Autodesk Inventor part; units mm, degrees
ref_plane "YZ Plane" through (0, 0, 0) normal (1, 0, 0) x (0, 1, 0)
ref_plane "XZ Plane" through (0, 0, 0) normal (0, 1, 0) x (-1, 0, 0)
ref_plane "XY Plane" through (0, 0, 0) normal (0, 0, 1) x (1, 0, 0)
sketch "Sketch1" plane through (0, 0, 0) normal (0, 0, 1) x (1, 0, 0)
  line L0 (0, 10.2918) -> (25, 10.2918)
  line L1 (25, 10.2918) -> (25, 0.2918)
  line L2 (25, 0.2918) -> (0, 0.2918)
  line L3 (0, 0.2918) -> (0, 10.2918)
  line L4 (2, 0.2918) -> (10, 0.2918)
  line L5 (10, 0.2918) -> (10, 3.2918)
  line L6 (10, 3.2918) -> (2, 3.2918)
  line L7 (2, 3.2918) -> (2, 0.2918)
  line L8 (0, 5.2918) -> (25, 5.2918) construction
  line L9 (12.5, 10.2918) -> (12.5, 0.2918) construction
  line L10 (23, 0.2918) -> (15, 0.2918)
  line L11 (15, 0.2918) -> (15, 3.2918)
  line L12 (15, 3.2918) -> (23, 3.2918)
  line L13 (23, 3.2918) -> (23, 0.2918)
  line L14 (2, 10.2918) -> (10, 10.2918)
  line L15 (10, 10.2918) -> (10, 7.2918)
  line L16 (10, 7.2918) -> (2, 7.2918)
  line L17 (2, 7.2918) -> (2, 10.2918)
  line L18 (23, 10.2918) -> (15, 10.2918)
  line L19 (15, 10.2918) -> (15, 7.2918)
  line L20 (15, 7.2918) -> (23, 7.2918)
  line L21 (23, 7.2918) -> (23, 10.2918)
  point P0 (0, 0)
  dimension "d0" = 25
  dimension "d1" = 10
  dimension "d2" = 3
  dimension "d3" = 2
  dimension "d4" = 8
extrude "Extrusion1" add sketch "Sketch1" along normal blind 3 contours L0 L17 L16 L15 L19 L20 L21 L1 L2 L13 L12 L11 L5 L6 L7 L3
properties part number "techoProctetorSensorHal"
Geometry check sheet. Reference: the model listing, model coordinates, mm. A direction names the side the tool comes from. Give positions to 0.01 mm unless a question says otherwise; leave off trailing zeros. Loops run counter-clockwise (first coordinate to the right, second up) from the corner with the lowest first, then second, coordinate; pieces in that order, holes last. Notation, with made-up numbers: M 22.5,11.25 L 37.5,11.25 A28 ccw 37.5,39.25 Z; hole C 11,78 d7. An arc over 180 degrees is marked long. Write each question's results on one line, items separated by ' | '.
1) Thickness scan on line 1 (X direction, y = 7.5, z = 2.7); line 2 (Y direction, x = 18, z = 2.05). Record the ranges inside material, lowest first.
Answers follow:
line 1: 0 to 2, 10 to 15, 23 to 25 | line 2: 3.29 to 7.29
2) Section check C-C, the plane x = 16. Record the boundary of the cut face in (y, z), plus the area to 3 significant figures.
Answers follow:
outline: M 3.29,0 L 7.29,0 L 7.29,3 L 3.29,3 Z | area: 12.0 mm2
3) Section check B-B, the plane z = 1.5. Record the boundary of the cut face in (x, y), plus the area to 3 significant figures.
Answers follow:
outline: M 0,0.29 L 2,0.29 L 2,3.29 L 10,3.29 L 10,0.29 L 15,0.29 L 15,3.29 L 23,3.29 L 23,0.29 L 25,0.29 L 25,10.29 L 23,10.29 L 23,7.29 L 15,7.29 L 15,10.29 L 10,10.29 L 10,7.29 L 2,7.29 L 2,10.29 L 0,10.29 Z | area: 154 mm2
4) Tool access check on faces 4 (the face through (23, 9, 1)), 5 (the face through (24, 10.292, 1)), 6 (the face through (10, 2, 1)). Record the directions out of +Z, -Z, +X, -X, +Y, -Y that give a thin tool (end or side, any length) a straight path to the whole face; none if there is none.
Answers follow:
face 4: +Z, -Z, +Y | face 5: +Z, -Z, +X, -X, +Y | face 6: +Z, -Z, -Y
5) Gauge pin test, flat ends, axial feed: pin 1 (0.9 mm diameter, centred on x = 21, z = 1, fed in from -Y); pin 2 (0.9 mm diameter, centred on x = 5, z = 1, fed in from +Y). Record the tip position at first contact, or that the pin passes through.
Answers follow:
pin 1: y = 3.29 | pin 2: y = 7.29
6) Release check for a two-part mould opening along X. For faces 1 (the face through (25, 5, 1)), 2 (the face through (10, 9, 1)), 3 (the face through (1, 10.292, 1)) record: +X half, -X half, draft (parallel to the pull), parting line (faces both ways), or undercut.
Answers follow:
face 1: +X half | face 2: undercut | face 3: draft
7) Section check A-A, the plane y = 8.5. Record the boundary of the cut face in (x, z), plus the area to 3 significant figures.
Answers follow:
outline: M 0,0 L 2,0 L 2,3 L 0,3 Z; M 10,0 L 15,0 L 15,3 L 10,3 Z; M 23,0 L 25,0 L 25,3 L 23,3 Z | area: 27.0 mm2
